The drawing under review shows one solid part. Ordinate dimensions are in mm from its lowest x, y, z. A direction names the side the tool comes from. Coordinates: 2 decimals unless noted, no trailing zeros. Write each loop counter-clockwise with the first axis right and the second up, starting at its lowest first coordinate (ties: lowest second). Pieces come first, ordered by that corner, then holes. Notation, with made-up numbers: (-14, -38.75) -> (17, -38.75) arc R21 cw to (17, -23.75) -> close; hole circle Ø1 at (39, -1.5). An arc over 180 degrees is marked (long way). One line per item, written item: value. Start each with the question number.
1) Add section C-C (x = 9). State the section outline as (y, z) points.
2) Add section A-A (x = 15.2). State the section outline as (y, z) points.
3) Add section D-D (z = 11.5). State the section outline as (x, y) points.
4) For pin 1 Ø1.5 at (x, z) = (18, 10.5) entering from +Y; pin 2 Ø6 at (y, z) = (14.5, 19) entering from +X; pin 3 Ø4 at (x, z) = (12, 5) entering from -Y, all flat-tipped, find the tip position at first contact; note any pin that passes through.
5) Add section B-B (y = 11). State the section outline as (x, z) points, and give its area (3 significant figures).
6) For probe 1 along Y at (x, z) = (15.2, 22.75); probe 2 along X at (y, z) = (17.5, 12.5); probe 3 along Z at (x, y) = (3.5, 19.5), list the stretches that pass through material, from the lowest coordinate up. Write a range as from..to.
7) Machinability: for the marked faces 1 and 2, which of the approach directions +Z, -Z, +X, -X, +Y, -Y give a long, thin tool a straight path to every point of the face, cutting with its end or side? Answer none if there is none.
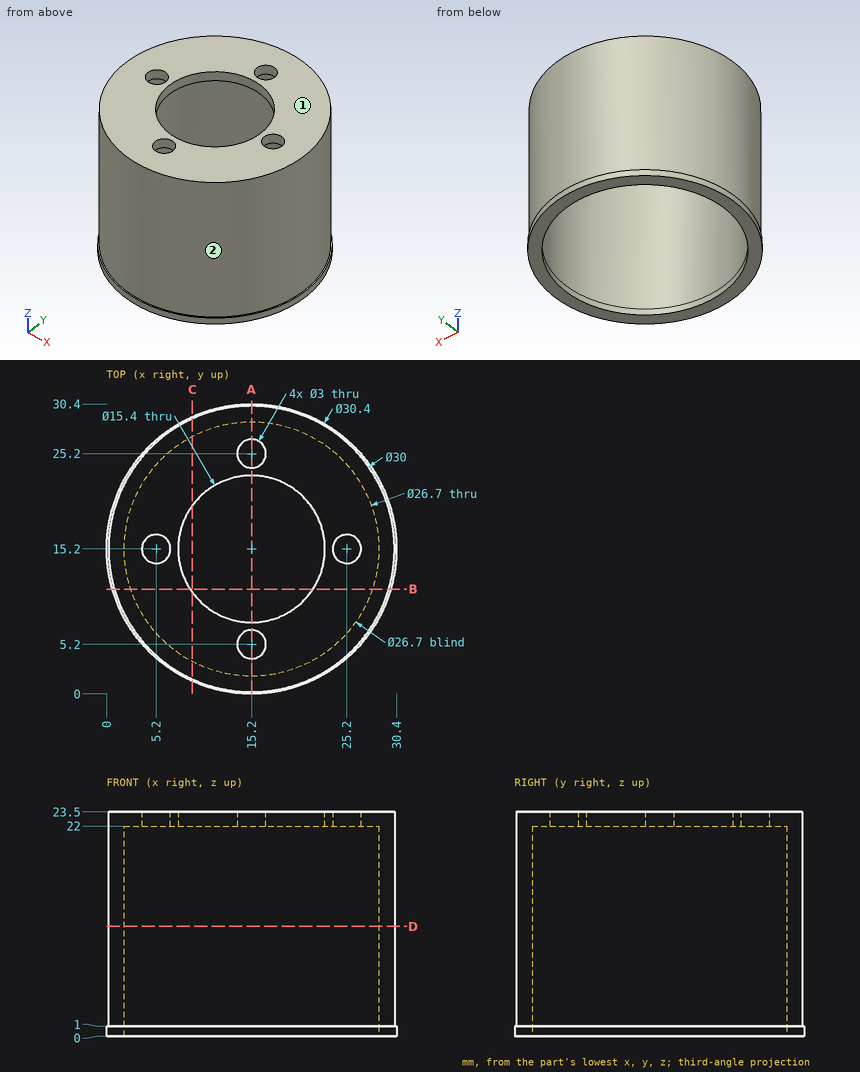
Numbers:
1. outline: (1.32, 0) -> (3.38, 0) -> (3.38, 22) -> (10.63, 22) -> (10.63, 23.5) -> (1.54, 23.5) -> (1.54, 1) -> (1.32, 1) -> close; (19.77, 22) -> (27.02, 22) -> (27.02, 0) -> (29.08, 0) -> (29.08, 1) -> (28.86, 1) -> (28.86, 23.5) -> (19.77, 23.5) -> close
2. outline: (0, 0) -> (1.85, 0) -> (1.85, 22) -> (3.7, 22) -> (3.7, 23.5) -> (0.2, 23.5) -> (0.2, 1) -> (0, 1) -> close; (6.7, 22) -> (7.5, 22) -> (7.5, 23.5) -> (6.7, 23.5) -> close; (22.9, 22) -> (23.7, 22) -> (23.7, 23.5) -> (22.9, 23.5) -> close; (26.7, 22) -> (28.55, 22) -> (28.55, 0) -> (30.4, 0) -> (30.4, 1) -> (30.2, 1) -> (30.2, 23.5) -> (26.7, 23.5) -> close
3. outline: circle Ø30 at (15.2, 15.2); hole circle Ø26.7 at (15.2, 15.2)
4. pin 1: y = 30.06
4. pin 2: x = 30.2
4. pin 3: y = 0.25
5. outline: (0.59, 0) -> (2.53, 0) -> (2.53, 22) -> (8.75, 22) -> (8.75, 23.5) -> (0.8, 23.5) -> (0.8, 1) -> (0.59, 1) -> close; (21.65, 22) -> (27.87, 22) -> (27.87, 0) -> (29.81, 0) -> (29.81, 1) -> (29.6, 1) -> (29.6, 23.5) -> (21.65, 23.5) -> close
5. area: 100 mm²
6. probe 1: 0.2..3.7, 6.7..7.5, 22.9..23.7, 26.7..30.2
6. probe 2: 0.38..2.05, 28.35..30.02
6. probe 3: 22..23.5
7. face 1: +Z, +X, -X, +Y, -Y
7. face 2: +Z
